Build history of the part. All positions in model axes, mm. A direction names the side the tool comes from. Round coordinates to 2 decimals unless told otherwise and drop trailing zeros. Order: outer loops, then holes, each group sorted by start corner. A loop starts at its lowest first (then second) coordinate and runs counter-clockwise, first axis right, second up. Notation, with made-up numbers: (-1.75, 49.5) -> (20.25, 49.5) arc R22 cw to (20.25, 66.5) -> close; hole circle Ø8 at (-35.5, 11). An arc over 180 degrees is marked (long way). Write item = value, one per line.
Autodesk Inventor part; units mm, degrees
ref_plane "YZ Plane" through (0, 0, 0) normal (1, 0, 0) x (0, 1, 0)
ref_plane "XZ Plane" through (0, 0, 0) normal (0, 1, 0) x (-1, 0, 0)
ref_plane "XY Plane" through (0, 0, 0) normal (0, 0, 1) x (1, 0, 0)
sketch "Sketch1" plane through (0, 0, 0) normal (0, 1, 0) x (-1, 0, 0)
  circle A0 centre (0, 0) radius 2.625
  dimension "d0" = 5.25
extrude "Extrusion1" add sketch "Sketch1" along normal blind 65
sketch "Sketch2" plane through (0, 65, 0) normal (0, 1, 0) x (1, 0, 0)
  circle A0 centre (0, 0) radius 2.625
  line L0 (-2.625, 0) -> (2.625, 0)
  arc A1 (2.625, 0) -> (-2.625, 0) centre (0, 0) ccw
extrude "Extrusion2" cut sketch "Sketch2" against normal blind 4 contours L0 A0 picked at (0.6549, 0.5802)
sketch "Sketch3" plane through (0, 0, 0) normal (0, -1, 0) x (1, 0, 0)
  arc A0 (2.625, 0) -> (-2.625, 0) centre (0, 0) ccw
  line L0 (2.625, 0) -> (-2.625, 0)
  line L1 (2.625, 0) -> (-2.625, 0)
  arc A1 (2.625, 0) -> (-2.625, 0) centre (0, 0) ccw
extrude "Extrusion3" cut sketch "Sketch3" against normal blind 6.2
properties part number "Twist_Rod"
Q1. Cut at C-C, the plane z = -0.95. List the corners of the cut face in (x, y).
Check values:
outline = (-2.45, 0) -> (2.45, 0) -> (2.45, 61) -> (-2.45, 61) -> close
Q2. Flat gauge pins, fed straight in: pin 1 (0.8 mm diameter, centred on x = 0, z = 1, fed in from -Y); pin 2 (1 mm diameter, centred on x = 2, y = 37, fed in from +Z); pin 3 (1.2 mm diameter, centred on x = -1, y = 62.5, fed in from -Z). Where does each tip first touch, or does it go through?
Check values:
pin_1 = 6.2
pin_2 = 2.15
pin_3 = 0
Q3. Cut at B-B, the plane y = 7. List the corners of the cut face in (x, z) (3 decimals), and give its area (3 significant figures).
Check values:
outline = circle Ø5.25 at (0, 0)
area = 21.6 mm²
Q4. Cut at A-A, the plane x = 0. List the corners of the cut face in (y, z) (3 decimals).
Check values:
outline = (0, -2.625) -> (61, -2.625) -> (61, 0) -> (65, 0) -> (65, 2.625) -> (6.2, 2.625) -> (6.2, 0) -> (0, 0) -> close
Q5. Which spindle directions (+Z, -Z, +X, -X, +Y, -Y) get a long thin tool onto all of the face, cutting with end or side? Do faces 1 (the face through (0, 65, 1)), 2 (the face through (0, 63, 0)), 3 (the face through (0, 3, 0)). Say none if no direction does.
Check values:
face_1 = +Z, -Z, +X, -X, +Y
face_2 = -Z, +X, -X, +Y
face_3 = +Z, +X, -X, -Y
Q6. Cut at D-D, the plane z = 1.95. List the corners of the cut face in (x, y).
Check values:
outline = (-1.76, 6.2) -> (1.76, 6.2) -> (1.76, 65) -> (-1.76, 65) -> close
Q7. Probe probe 1 along Y at (x, z) = (-0.5, 1.2); probe 2 along X at (y, z) = (28, -0.2). List the from-to ranges inside material, lowest first.
Check values:
probe_1 = 6.2 to 65
probe_2 = -2.62 to 2.62
